Source: CAD feature listing. Evaluate the final solid. Frame: model axes, mm. A direction names the side the tool comes from. Round coordinates to 2 decimals unless told otherwise and drop trailing zeros. Loops run counter-clockwise (first coordinate to the right, second up) from the corner with the lowest first, then second, coordinate; pieces in that order, holes last.
(1) Set-up query: faces 1 (the flat face through (0, 8, 8)), 2 (the flat face through (0, -8, -8)), 3 (the cylindrical face through (9.86, -11.08, -4.48)). Return all of +Z, -Z, +X, -X, +Y, -Y with unobstructed straight access to the full face (end or side cutting, diameter ignored); none if empty.
(2) First-contact query: pin 1 Ø8 at (x, z) = (0, -11) entering from +Y; pin 2 Ø12 at (x, y) = (13.5, 0.5) entering from +Z; pin 3 Ø1.7 at (y, z) = (2.5, -11.5) entering from -X. Flat tips, straight axial feed; report the tip coordinate or a pass-through.
(3) Mould query, pull axis Z, two halves, no side actions, for faces 4 (the cylindrical face through (9.86, -9.384, -7.297)), 5 (the flat face through (0, -8, 8)). Classes: pulls with the +Z half, pulls with the -Z half, needs draft (parallel to the pull), parting line crosses it, or undercut.
(4) Material intervals for probe 1 along Y at (x, z) = (5, 8.5); probe 2 along Z at (x, y) = (7, -9); probe 3 along Y at (x, z) = (-5, 0), sorted ascending.
(5) Section A-A, the plane z = 0. Return the cut outline in (x, y).
(6) Section D-D, the plane y = -2.75. Return the cut outline in (x, z).
(7) Section C-C, the plane x = -4. Return the cut outline in (y, z).
```python
from build123d import *
from build123d.topology import SkipClean

# Parameters (mm, degrees)
BASPROSKE_W      = 20
BASPROSKE_H      = 14
TOOTHCUT_DEPTH   = 29.142494559
TEETHCUTS_COUNT  = 12
TEETHCUTS_ANGLE  = 330
HUBNEAONESKE_R   = 9.499
HUBNEARONE_DEPTH = 10.0000508
BORSKE_R         = 0.4
BORE_DEPTH       = 30.0000508


with BuildPart() as part:
    # BasProSke → Base-Revolve (revolve)
    with BuildSketch(Plane(origin=(0, 0, 0), x_dir=(1, 0, 0), z_dir=(0, 1, 0)), mode=Mode.PRIVATE) as base_revolve_sk:
        with Locations((10, 7)):
            Rectangle(BASPROSKE_W, BASPROSKE_H)
    revolve(base_revolve_sk.sketch.rotate(Axis((-10, 0, 0), (1, 0, 0)), 180), axis=Axis((-10, 0, 0), (1, 0, 0)))

    # TooCutSke → ToothCut (cut, through all)
    with BuildSketch(Plane(origin=(0, 0, 0), x_dir=(0, 0, -1), z_dir=(1, 0, 0))):
        with BuildLine():
            ThreePointArc((1.111908866, 9.433698091), (0, 9.499), (-1.111908866, 9.433698091))
            ThreePointArc((-1.111908866, 9.433698091), (-1.651516138, 11.821129337), (-3.298149691, 13.632096456))
            ThreePointArc((-3.298149691, 13.632096456), (0, 14.0254), (3.298149691, 13.632096456))
            ThreePointArc((3.298149691, 13.632096456), (1.651516138, 11.821129337), (1.111908866, 9.433698091))
        make_face()
    toothcut = extrude(amount=TOOTHCUT_DEPTH, mode=Mode.SUBTRACT)

    # TeethCuts: ToothCut ×12 about axis
    teethcuts_axis = Axis((-10, 0, 0), (1, 0, 0))
    for i in range(1, TEETHCUTS_COUNT):
        add(toothcut.rotate(teethcuts_axis, i * TEETHCUTS_ANGLE / (TEETHCUTS_COUNT - 1)), mode=Mode.SUBTRACT)

    # HubNeaOneSke → HubNearOne (add)
    with SkipClean():  # the faces are left unmerged after this step: merging them gives an invalid solid
        with BuildSketch(Plane.ZY):
            Circle(HUBNEAONESKE_R)
        extrude(amount=HUBNEARONE_DEPTH)

    # BorSke → Bore (cut, symmetric)
    with SkipClean():  # the faces are left unmerged after this step: merging them gives an invalid solid
        with BuildSketch(Plane(origin=(0, 0, 0), x_dir=(0, 0, -1), z_dir=(1, 0, 0))):
            with Locations(Location((0, 0, 0), (0, 0, 180))):
                Circle(BORSKE_R)
        extrude(amount=BORE_DEPTH, both=True, mode=Mode.SUBTRACT)


solid = part.part
```
Output values:
1. face 1: +Z, -X, +Y
1. face 2: -Z, -X, -Y
1. face 3: +X, -X
2. pin 1: stops at y = 10.15
2. pin 2: stops at z = 13.61
2. pin 3: stops at x = 0
3. face 4: undercut
3. face 5: needs draft
4. probe 1: y = -9.95 to -6.29, -4.24 to 4.24, 6.29 to 9.95
4. probe 2: z = -10.07 to -6.79, -3.91 to 3.91, 6.79 to 10.07
4. probe 3: y = -9.5 to -0.4, 0.4 to 9.5
5. outline: (-10, -9.5) - (20, -9.5) - (20, -0.4) - (-10, -0.4) - close; (-10, 0.4) - (20, 0.4) - (20, 9.5) - (-10, 9.5) - close
6. outline: (-10, -9.09) - (0, -9.09) - (0, -13.22) - (20, -13.22) - (20, 13.22) - (0, 13.22) - (0, 9.09) - (-10, 9.09) - close
7. outline: circle Ø19 at (0, 0); hole circle Ø0.8 at (0, 0)
